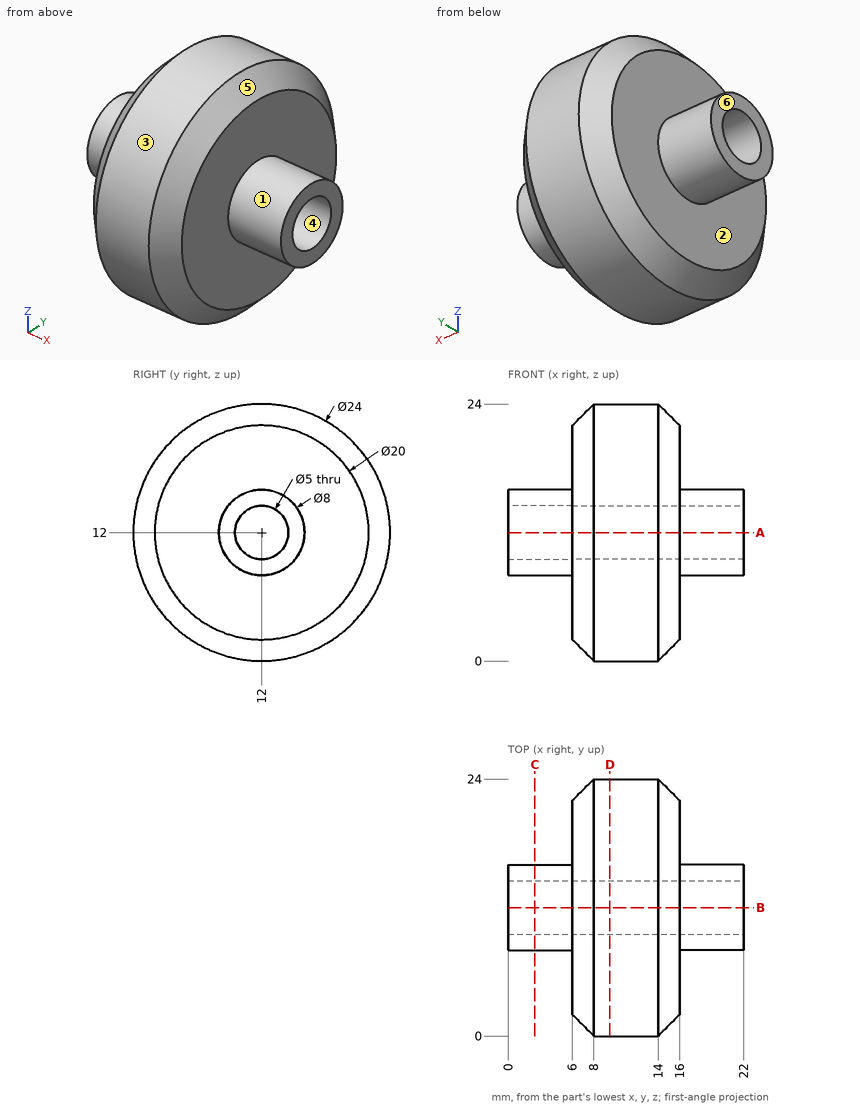
Could you check a few things on this drawing? It's one solid part, dimensions in mm from its lowest x, y, z. A direction names the side the tool comes from. Give positions to 0.01 mm unless a question says otherwise; leave off trailing zeros. Order: outer loops, then holes, each group sorted by start corner. A loop starts at its lowest first (then second) coordinate and runs counter-clockwise, first axis right, second up. Notation, with made-up numbers: (-21, 36.5) -> (-1, 36.5) arc R30 cw to (-1, 71.5) -> close; hole circle Ø11 at (73, 86.25). An arc over 180 degrees is marked (long way). Answer in a Markdown table with one row per item. Add a question column.
Item 1: We'd pull the mould along Z, two halves only. Please class the marked faces 4, 5 and 6: pulls with the +Z half, pulls with the -Z half, needs draft (parallel to the pull), parting line crosses it, or undercut.
Item 2: For the marked faces 1, 2 and 3, which set-ups out of +Z, -Z, +X, -X, +Y, -Y let a thin tool reach every point of the face, with its end or its side?
Item 3: I'm going to push flat-ended pins straight in: P1, Ø1.5, axis at x = 7, y = 5.5, coming from the +Z side; P2, Ø12, axis at y = 21.5, z = 8.5, coming from the -X side; P3, Ø2, axis at y = 21, z = 15, coming from the +X side. Where does each tip first touch, or does it pass through?
Item 4: Imagine slicing it at A-A (z = 12). List the corners of the cut face in (x, y) for me.
Item 5: Imagine slicing it at D-D (x = 9.5). List the corners of the cut face in (y, z) for me, and give its area (3 significant figures).
Item 6: Please list where these lines run through material, in increasing order: probe 1 along X at (y, z) = (19, 17); probe 2 along Z at (x, y) = (9.5, 12); probe 3 along Y at (x, z) = (8.75, 11.75).
Item 7: Imagine slicing it at C-C (x = 2.5). List the corners of the cut face in (y, z) for me.
Result:
| question | item | result |
|---|---|---|
| 1 | face 4 | undercut |
| 1 | face 5 | parting line crosses it |
| 1 | face 6 | needs draft |
| 2 | face 1 | +X |
| 2 | face 2 | -X |
| 2 | face 3 | +X, -X |
| 3 | P1 | z = 21.91 |
| 3 | P2 | x = 6 |
| 3 | P3 | x = 16 |
| 4 | outline | (0, 8) -> (6, 8) -> (6, 2) -> (8, 0) -> (14, 0) -> (16, 2) -> (16, 8) -> (22, 8) -> (22, 9.5) -> (0, 9.5) -> close; (0, 14.5) -> (22, 14.5) -> (22, 16) -> (16, 16) -> (16, 22) -> (14, 24) -> (8, 24) -> (6, 22) -> (6, 16) -> (0, 16) -> close |
| 5 | outline | circle Ø24 at (12, 12); hole circle Ø5 at (12, 12) |
| 5 | area | 433 mm2 |
| 6 | probe 1 | 6 to 16 |
| 6 | probe 2 | 0 to 9.5, 14.5 to 24 |
| 6 | probe 3 | 0 to 9.51, 14.49 to 24 |
| 7 | outline | circle Ø8 at (12, 12); hole circle Ø5 at (12, 12) |
